```python
from build123d import *

# Parameters (mm, degrees)
BOSS_EXTRUDE1_DEPTH = 47.5
CUT_EXTRUDE1_START  = 48
SKETCH1_3_R         = 2.5
CUT_EXTRUDE1_DEPTH  = 14
CUT_EXTRUDE2_START  = -34
SKETCH1_4_R         = 2.5
CUT_EXTRUDE2_DEPTH  = 14


with BuildPart() as part:
    # Sketch1 → Boss-Extrude1 (new, symmetric)
    with BuildSketch(Plane(origin=(0, 0, 0), x_dir=(1, 0, 0), z_dir=(0, 1, 0))):
        Polygon((4.052090098, 2.216731642), (0.106299134, 4.617578784), (-3.945790964, 2.400847142), (-4.052090098, -2.216731642), (-0.106299134, -4.617578784), (3.945790964, -2.400847142), align=None)
    extrude(amount=BOSS_EXTRUDE1_DEPTH, both=True)

    # Sketch1<3> → Cut-Extrude1 (cut)
    with BuildSketch(Plane(origin=(0, 0, 0), x_dir=(1, 0, 0), z_dir=(0, 1, 0)).offset(CUT_EXTRUDE1_START)):
        with Locations(Location((0, 0, 0), (0, 0, 270))):
            Circle(SKETCH1_3_R)
    extrude(amount=-CUT_EXTRUDE1_DEPTH, mode=Mode.SUBTRACT)

    # Sketch1<4> → Cut-Extrude2 (cut)
    with BuildSketch(Plane(origin=(0, 0, 0), x_dir=(1, 0, 0), z_dir=(0, 1, 0)).offset(CUT_EXTRUDE2_START)):
        with Locations(Location((0, 0, 0), (0, 0, 270))):
            Circle(SKETCH1_4_R)
    extrude(amount=-CUT_EXTRUDE2_DEPTH, mode=Mode.SUBTRACT)


solid = part.part
```
For this review, take the finished solid that the model builds, in its own axes (mm). A direction names the side the tool comes from. Coordinates: 2 decimals unless noted, no trailing zeros. Write each loop counter-clockwise with the first axis right and the second up, starting at its lowest first coordinate (ties: lowest second). Pieces come first, ordered by that corner, then holes. Notation, with made-up numbers: (69.5, 33) - (116.5, 33) arc R33 cw to (116.5, 65) - close; hole circle Ø11 at (2.5, 31). An arc over 180 degrees is marked (long way). Answer in a Markdown table with one row per item. Add a question column.
Q1. We need section B-B, the plane y = -13. State the section outline as (x, z) points.
Q2. Draft analysis for pull direction Z (two halves, no side actions). For faces 4 (the flat face through (2, -47.5, 2)), 5 (the flat face through (1.891, 0.665, 3.525)), 6 (the flat face through (0, 34, 0)), state which applies: +Z half, -Z half, draft (parallel to the pull), parting line (faces both ways), or undercut.
Q3. We need section A-A, the plane y = 40. State the section outline as (x, z) points.
Q4. Tool access review of faces 1 (the flat face through (-2.11, 0.66, 3.4)), 2 (the cylindrical face through (-2.44, 40.84, -0.54)), 3 (the cylindrical face through (-2.44, -40.66, -0.54)): name each direction out of +Z, -Z, +X, -X, +Y, -Y from which nothing blocks a thin tool from reaching the whole face with its end or side.
Q5. We need section D-D, the plane x = 1.5. State the section outline as (y, z) points, and give its area (3 significant figures).
Q6. We need section C-C, the plane z = 1. State the section outline as (x, y) points, and give its area (3 significant figures).
Q7. For P1, Ø1.5, axis at y = 33, z = 0, coming from the -X side; P2, Ø1.5, axis at x = 1, y = -25, coming from the -Z side; P3, Ø4.5, axis at x = 0, z = 0, coming from the -Y side, all flat-tipped, find the tip position at first contact; note any pin that passes through.
Q8. For probe 1 along Y at (x, z) = (0.25, 0.5); probe 2 along X at (y, z) = (44.75, 0); probe 3 along Z at (x, y) = (0.5, -39), list the stretches that pass through material, from the lowest coordinate up.
Answer list:
| question | item | result |
|---|---|---|
| 1 | outline | (-4.05, 2.22) - (-3.95, -2.4) - (0.11, -4.62) - (4.05, -2.22) - (3.95, 2.4) - (-0.11, 4.62) - close |
| 2 | face 4 | draft |
| 2 | face 5 | +Z half |
| 2 | face 6 | undercut |
| 3 | outline | (-4.05, 2.22) - (-3.95, -2.4) - (0.11, -4.62) - (4.05, -2.22) - (3.95, 2.4) - (-0.11, 4.62) - close; hole circle Ø5 at (0, 0) |
| 4 | face 1 | +Z, -X, +Y, -Y |
| 4 | face 2 | +Y |
| 4 | face 3 | -Y |
| 5 | outline | (-47.5, -3.77) - (47.5, -3.77) - (47.5, -2) - (34, -2) - (34, 2) - (47.5, 2) - (47.5, 3.74) - (-47.5, 3.74) - (-47.5, 2) - (-34, 2) - (-34, -2) - (-47.5, -2) - close |
| 5 | area | 605 mm2 |
| 6 | outline | (-4.02, -47.5) - (-2.29, -47.5) - (-2.29, -34) - (2.29, -34) - (2.29, -47.5) - (3.98, -47.5) - (3.98, 47.5) - (2.29, 47.5) - (2.29, 34) - (-2.29, 34) - (-2.29, 47.5) - (-4.02, 47.5) - close |
| 6 | area | 636 mm2 |
| 7 | P1 | stops at x = -4.02 |
| 7 | P2 | stops at z = -4.53 |
| 7 | P3 | stops at y = -34 |
| 8 | probe 1 | y = -34 to 34 |
| 8 | probe 2 | x = -4 to -2.5, 2.5 to 4 |
| 8 | probe 3 | z = -4.38 to -2.45, 2.45 to 4.29 |
